Here's how the part is built. I have some questions about the finished solid (model axes, mm). Face numbers are marked on the shaded views. Round coordinates to 2 decimals unless told otherwise and drop trailing zeros. Loops run counter-clockwise (first coordinate to the right, second up) from the corner with the lowest first, then second, coordinate; pieces in that order, holes last. Notation, with made-up numbers: M -29,-16 L -21,-16 A24 cw -21,14 Z; hole C -17,-15 d9. An arc over 180 degrees is marked long. Answer as a JSON object with one key per item and string values.
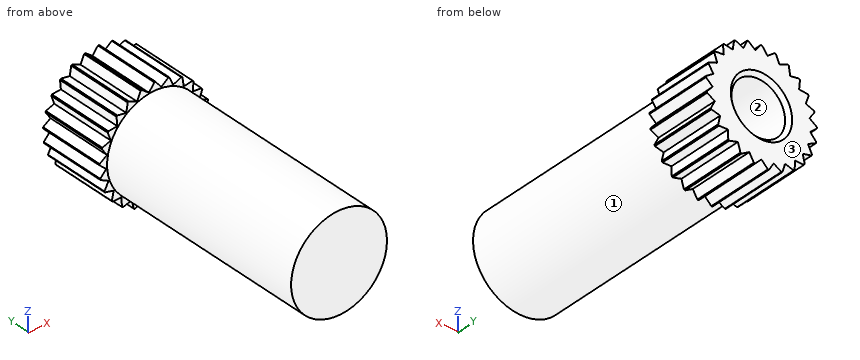
from build123d import *

# Parameters (mm, degrees)
SKETCH_1_R                  = 2.9
EXTRUDE_1_DEPTH             = 3.5
SKETCH_2_R                  = 2.5
EXTRUDE_2_DEPTH             = 11.4
CUT_EXTRUDE_1_DEPTH         = 4
HOLE_WIZARD_M32_D           = 2.8
HOLE_WIZARD_M32_DEPTH       = 6.9
HOLE_WIZARD_M32_CSINK_D     = 3.2
HOLE_WIZARD_M32_CSINK_ANGLE = 90
HOLE_WIZARD_M32_TIP         = 1.4


with BuildPart() as part:
    # Эскиз1 → Бобышка-Вытянуть1 (new body)
    with BuildSketch(Plane(origin=(0, 0, 0), x_dir=(1, 0, 0), z_dir=(0, 1, 0))):
        Circle(SKETCH_1_R)
    extrude(amount=EXTRUDE_1_DEPTH)

    # Эскиз2 → Бобышка-Вытянуть2 (add)
    with BuildSketch(Plane.XZ):
        Circle(SKETCH_2_R)
    extrude(amount=EXTRUDE_2_DEPTH)

    # Эскиз3 → Вырез-Вытянуть1 (cut)
    with BuildSketch(Plane(origin=(0, 3.5, 0), x_dir=(1, 0, 0), z_dir=(0, 1, 0))):
        Polygon((0, 2.55), (-0.366495157, 2.916495157), (0.366495157, 2.916495157), align=None)
        Polygon((0.634159212, 2.469887061), (0.370321814, 2.916011738), (1.080283889, 2.733724459), align=None)
        Polygon((1.228471869, 2.234582034), (1.083870103, 2.732304577), (1.726194412, 2.3791838), align=None)
        Polygon((1.74559512, 1.85887), (1.729314848, 2.37691667), (2.263641791, 1.875150272), align=None)
        Polygon((2.15303621, 1.366358327), (2.26610038, 1.872178348), (2.658856231, 1.253294157), align=None)
        Polygon((2.425194117, 0.787993336), (2.660498492, 1.249804175), (2.887004956, 0.55268896), align=None)
        Polygon((2.544968157, 0.160115825), (2.887727699, 0.548900209), (2.933752541, -0.182643716), align=None)
        Polygon((2.504832489, -0.477822352), (2.933510354, -0.186493176), (2.796161665, -0.906500217), align=None)
        Polygon((2.307308984, -1.085737193), (2.794969765, -0.910168509), (2.482877668, -1.573397974), align=None)
        Polygon((1.964808769, -1.625431174), (2.480810946, -1.576654607), (2.013585336, -2.141433351), align=None)
        Polygon((1.498852393, -2.062993336), (2.010773652, -2.144073698), (1.417772031, -2.574914594), align=None)
        Polygon((0.938717609, -2.370930039), (1.414392054, -2.576772752), (0.732874896, -2.846604484), align=None)
        Polygon((0.319599746, -2.529892488), (0.729139002, -2.847563698), (0.001928536, -2.939431745), align=None)
        Polygon((-0.319599746, -2.529892488), (-0.001928536, -2.939431745), (-0.729139002, -2.847563698), align=None)
        Polygon((-0.938717609, -2.370930039), (-0.732874896, -2.846604484), (-1.414392054, -2.576772752), align=None)
        Polygon((-1.498852393, -2.062993336), (-1.417772031, -2.574914594), (-2.010773652, -2.144073698), align=None)
        Polygon((-1.964808769, -1.625431174), (-2.013585336, -2.141433351), (-2.480810946, -1.576654607), align=None)
        Polygon((-2.307308984, -1.085737193), (-2.482877668, -1.573397974), (-2.794969765, -0.910168509), align=None)
        Polygon((-2.504832489, -0.477822352), (-2.796161665, -0.906500217), (-2.933510354, -0.186493176), align=None)
        Polygon((-2.544968157, 0.160115825), (-2.933752541, -0.182643716), (-2.887727699, 0.548900209), align=None)
        Polygon((-2.425194117, 0.787993336), (-2.887004956, 0.55268896), (-2.660498492, 1.249804175), align=None)
        Polygon((-2.15303621, 1.366358327), (-2.658856231, 1.253294157), (-2.26610038, 1.872178348), align=None)
        Polygon((-1.74559512, 1.85887), (-2.263641791, 1.875150272), (-1.729314848, 2.37691667), align=None)
        Polygon((-1.228471869, 2.234582034), (-1.726194412, 2.3791838), (-1.083870103, 2.732304577), align=None)
        Polygon((-0.634159212, 2.469887061), (-1.080283889, 2.733724459), (-0.370321814, 2.916011738), align=None)
    extrude(amount=-CUT_EXTRUDE_1_DEPTH, mode=Mode.SUBTRACT)

    # Сверло под метчик  спиральное M32
    with Locations(Plane(origin=(0, 3.5, 0), x_dir=(1, 0, 0), z_dir=(0, 1, 0))):
        with Locations((0, 0)):
            CounterSinkHole(HOLE_WIZARD_M32_D / 2, HOLE_WIZARD_M32_CSINK_D / 2, depth=HOLE_WIZARD_M32_DEPTH, counter_sink_angle=HOLE_WIZARD_M32_CSINK_ANGLE)
            with Locations((0, 0, -(HOLE_WIZARD_M32_DEPTH + HOLE_WIZARD_M32_TIP / 2))):  # 90° drill point
                Cone(0, HOLE_WIZARD_M32_D / 2, HOLE_WIZARD_M32_TIP, mode=Mode.SUBTRACT)


solid = part.part
Item 1: I want a section at A-A on y = -4.25. List the corners of the cut face in (x, z) for me, plus the area to 3 significant figures.
Solution:
{"outline": "C 0,0 d5; hole C 0,0 d1.1", "area": "18.7 mm2"}
Item 2: For P1, Ø1.5, axis at x = -2, z = -2, coming from the -Y side; P2, Ø1.5, axis at y = -5, z = -2, coming from the +X side; P3, Ø2, axis at x = -1, y = -4, coming from the -Z side; P4, Ø2, axis at y = -9, z = -0.5, coming from the -X side, each with a flat end and sliding along its axis, tell me the tip position at first contact or that it passes through.
Solution:
{"P1": "stops at y = -11.4", "P2": "stops at x = 2.17", "P3": "stops at z = -2.5", "P4": "stops at x = -2.5"}
Item 3: I want a section at B-B on y = -6.5. List the corners of the cut face in (x, z) for me, plus the area to 3 significant figures.
Solution:
{"outline": "C 0,0 d5", "area": "19.6 mm2"}
Item 4: If I drill on L1, parallel to Z at x = 0, y = -1; L2, parallel to X at y = -1.5, z = 0.9; L3, parallel to X at y = -6.25, z = -1.8, over which ranges is the centre line in solid material (lowest first)? Write a range as from..to.
Solution:
{"L1": "z = -2.5..-1.4, 1.4..2.5", "L2": "x = -2.33..-1.07, 1.07..2.33", "L3": "x = -1.73..1.73"}
Item 5: We'd pull the mould along X, two halves only. Please class the marked faces 1, 2 and 3: +X half, -X half, draft (parallel to the pull), parting line (faces both ways), or undercut.
Solution:
{"face 1": "parting line", "face 2": "undercut", "face 3": "draft"}
